Could you check a few things on this model? Use its own coordinates, in mm. Give positions to 0.01 mm unless a question says otherwise; leave off trailing zeros. Write each loop counter-clockwise with the first axis right and the second up, starting at its lowest first coordinate (ties: lowest second). Pieces come first, ordered by that corner, then holes. Notation, with made-up numbers: M 7.5,86.5 L 25.5,86.5 A16 cw 25.5,90.5 Z; hole C -27,86.25 d4. An arc over 180 degrees is marked long. Use one line per item in the form item = value.
from build123d import *

# Parameters (mm, degrees)
F0_R     = 12.7
F0_W     = 50.8
F0_H     = 12.7
F0_W_2   = 63.5
F1_DEPTH = 25.4


# Not quite as in the source:
# - a feature names something its author has since deleted; it is built from what else it names


with BuildPart() as f1:
    # F0 (on Top) → F1 (new body)
    with BuildSketch(Plane.XY):
        Polygon((-406.4, -964.5238018036), (-406.4, -1396.3238018036), (0, -1396.3238018036), (0, -964.5238018036), (254, -964.5238018036), (254, -454.310915063), (0, 127.6761981964), (-406.4, 127.6761981964), (-660.4, -454.310915063), (-660.4, -964.5238018036), align=None)
        with Locations((-203.2, -714.3330844099)):
            Circle(F0_R, mode=Mode.SUBTRACT)
        Polygon((-241.3, -316.8238018036), (-241.3, 76.8761981964), (-165.1, 76.8761981964), (-165.1, -316.8238018036), (-101.6, -316.8238018036), (0, -316.8238018036), (50.8, -316.8238018036), (50.8, -329.5238018036), (0, -329.5238018036), (-101.6, -329.5238018036), (-165.1, -329.5238018036), (-165.1, -354.9238018036), (-241.3, -354.9238018036), (-241.3, -329.5238018036), (-304.8, -329.5238018036), (-406.4, -329.5238018036), (-457.2, -329.5238018036), (-457.2, -316.8238018036), (-406.4, -316.8238018036), (-304.8, -316.8238018036), align=None, mode=Mode.SUBTRACT)
        with Locations((-431.8, -323.1738018036)):
            Rectangle(F0_W, F0_H)
        with Locations((-133.35, -323.1738018036)):
            Rectangle(F0_W_2, F0_H)
        with Locations((25.4, -323.1738018036)):
            Rectangle(F0_W, F0_H)
        with Locations((-273.05, -323.1738018036)):
            Rectangle(F0_W_2, F0_H)
    extrude(amount=F1_DEPTH)


solid = f1.part
1) I want a section at C-C, the plane y = -996.5. Please give me the cut outline in (x, z), plus the area to 3 significant figures.
Checked values:
outline = M -406.4,0 L 0,0 L 0,25.4 L -406.4,25.4 Z
area = 10,300 mm2
2) For pin 1 Ø10 at (y, z) = (-323, 17.5) entering from +X; pin 2 Ø7.5 at (x, z) = (93, 18) entering from -Y; pin 3 Ø12.5 at (y, z) = (-210, 12) entering from +X, each with a flat end and sliding along its axis, tell me the tip position at first contact or that it passes through.
Checked values:
pin_1 = 198.87
pin_2 = -964.52
pin_3 = 150.1
3) I want a section at A-A, the plane z = 14.5. Please give me the cut outline in (x, y).
Checked values:
outline = M -660.4,-964.52 L -406.4,-964.52 L -406.4,-1396.32 L 0,-1396.32 L 0,-964.52 L 254,-964.52 L 254,-454.31 L 0,127.68 L -406.4,127.68 L -660.4,-454.31 Z; hole M -406.4,-329.52 L -304.8,-329.52 L -304.8,-316.82 L -406.4,-316.82 Z; hole M -241.3,-354.92 L -165.1,-354.92 L -165.1,76.88 L -241.3,76.88 Z; hole C -203.2,-714.33 d25.4; hole M -101.6,-329.52 L 0,-329.52 L 0,-316.82 L -101.6,-316.82 Z
4) I want a section at B-B, the plane y = -268. Please give me the cut outline in (x, z).
Checked values:
outline = M -579.09,0 L -241.3,0 L -241.3,25.4 L -579.09,25.4 Z; M -165.1,0 L 172.69,0 L 172.69,25.4 L -165.1,25.4 Z
5) I want a section at D-D, the plane x = 40. Please give me the cut outline in (y, z).
Checked values:
outline = M -964.52,0 L 36.02,0 L 36.02,25.4 L -964.52,25.4 Z
6) If I drill on L1, parallel to Y at x = -203.2, z = 14; L2, parallel to X at y = -712.5, z = 19.5; L3, parallel to X at y = -1278.5, z = 3.5, over which ranges is the centre line in solid material (lowest first)?
Checked values:
L1 = -1396.32 to -727.03, -701.63 to -354.92, 76.88 to 127.68
L2 = -660.4 to -215.77, -190.63 to 254
L3 = -406.4 to 0
